```python
from build123d import *

# Parameters (mm, degrees)
F1_DEPTH = 67
F2_R     = 1.5
F3_DEPTH = 8
F4_R     = 1.875
F5_DEPTH = 9
F6_R     = 1.875
F7_DEPTH = 9
F8_R     = 1.875
F9_DEPTH = 9


# Not quite as in the source:
# - a feature names something its author has since deleted; it is built from what else it names


with BuildPart() as f1:
    # F0 (on Right) → F1 (new body)
    with BuildSketch(Plane.YZ):
        Polygon((14.9777059274, -37.1211464703), (14.9777059274, 53.8788535297), (8.9777059274, 53.8788535297), (8.9777059274, -31.1211464703), (5.4777059274, -31.1211464703), (5.4777059274, -16.1211464703), (-0.5222940726, -16.1211464703), (-0.5222940726, -37.1211464703), align=None)
    extrude(amount=F1_DEPTH)

    # F2 (on face) → F3 (join)
    with BuildSketch(Plane.YZ.offset(67)):
        with BuildLine():
            Line((11.9777059274, 43.8788535297), (11.9777059274, 45.3788535297))
            ThreePointArc((11.9777059274, 45.3788535297), (10.4777059274, 43.8788535297), (11.9777059274, 42.3788535297))
            Line((11.9777059274, 42.3788535297), (11.9777059274, 43.8788535297))
        make_face()
        with BuildLine():
            ThreePointArc((11.9777059274, 42.3788535297), (13.0383660992, 42.8181933579), (13.4777059274, 43.8788535297))
            ThreePointArc((13.4777059274, 43.8788535297), (13.0383660992, 44.9395137015), (11.9777059274, 45.3788535297))
            Line((11.9777059274, 45.3788535297), (11.9777059274, 43.8788535297))
            Line((11.9777059274, 43.8788535297), (11.9777059274, 42.3788535297))
        make_face()
        with BuildLine():
            ThreePointArc((13.4777059274, 23.8788535297), (13.0383660992, 24.9395137015), (11.9777059274, 25.3788535297))
            ThreePointArc((11.9777059274, 25.3788535297), (10.9170457557, 22.8181933579), (13.4777059274, 23.8788535297))
        make_face()
        with Locations((11.9777059274, -7.1211464703)):
            Circle(F2_R)
        with Locations((11.9777059274, -27.1211464703)):
            Circle(F2_R)
    extrude(amount=F3_DEPTH)

    # F4 (on face) → F5 (cut)
    with BuildSketch(Plane(origin=(0, 0, 0), x_dir=(0, -1, 0), z_dir=(-1, 0, 0))):
        with Locations((-18.4777059274, 23.8788535297)):
            Circle(F4_R)
        with Locations((-18.4777059274, 43.8788535297)):
            Circle(F4_R)
        with Locations((-18.4777059274, -7.1211464703)):
            Circle(F4_R)
        with Locations((-18.4777059274, -27.1211464703)):
            Circle(F4_R)
    extrude(amount=-F5_DEPTH, mode=Mode.SUBTRACT)

    # F6 (on face) → F7 (cut)
    with BuildSketch(Plane(origin=(0, 14.9777059274, 0), x_dir=(-1, 0, 0), z_dir=(0, 1, 0))):
        with Locations((-47, -34.1211464703)):
            Circle(F6_R)
        with Locations((-20, -34.1211464703)):
            Circle(F6_R)
    extrude(amount=-F7_DEPTH, mode=Mode.SUBTRACT)

    # F8 (on face) → F9 (cut)
    with BuildSketch(Plane(origin=(0, 0, 0), x_dir=(0, -1, 0), z_dir=(-1, 0, 0))):
        with BuildLine():
            ThreePointArc((-10.1027059274, 43.8788535297), (-10.6518807127, 45.2046787444), (-11.9777059274, 45.7538535297))
            Line((-11.9777059274, 45.7538535297), (-11.9777059274, 43.8788535297))
            Line((-11.9777059274, 43.8788535297), (-11.9777059274, 42.0038535297))
            ThreePointArc((-11.9777059274, 42.0038535297), (-10.6518807127, 42.553028315), (-10.1027059274, 43.8788535297))
        make_face()
        with BuildLine():
            ThreePointArc((-10.1027059274, 23.8788535297), (-10.6518807127, 25.2046787444), (-11.9777059274, 25.7538535297))
            ThreePointArc((-11.9777059274, 25.7538535297), (-13.3035311422, 22.553028315), (-10.1027059274, 23.8788535297))
        make_face()
        with BuildLine():
            Line((-11.9777059274, 43.8788535297), (-11.9777059274, 45.7538535297))
            ThreePointArc((-11.9777059274, 45.7538535297), (-13.8527059274, 43.8788535297), (-11.9777059274, 42.0038535297))
            Line((-11.9777059274, 42.0038535297), (-11.9777059274, 43.8788535297))
        make_face()
        with Locations((-11.9777059274, -27.1211464703)):
            Circle(F8_R)
        with Locations((-11.9777059274, -7.1211464703)):
            Circle(F8_R)
    extrude(amount=-F9_DEPTH, mode=Mode.SUBTRACT)


solid = f1.part
```
Geometry check sheet. Reference: the model listing, model coordinates, mm. A direction names the side the tool comes from. Give positions to 0.01 mm unless a question says otherwise; leave off trailing zeros. Order: outer loops, then holes, each group sorted by start corner. A loop starts at its lowest first (then second) coordinate and runs counter-clockwise, first axis right, second up. Notation, with made-up numbers: (-6.75, 57.5) - (29.25, 57.5) arc R18 ccw to (29.25, 63.5) - close; hole circle Ø8 at (17.25, 88.5). An arc over 180 degrees is marked (long way). Answer in a Markdown table with one row per item. Add a question column.
Q1. Cross-section at C-C, the plane x = 30. Enter the section's corners in (y, z).
Q2. Cross-section at D-D, the plane z = 21. Enter the section's corners in (x, y), then the cut area to 3 significant figures.
Q3. Tool access check on faces 4 (the flat face through (33, 3, -16.121)), 5 (the cylindrical face through (70.94, 12.67, -8.45)), 6 (the flat face through (33, 7, -31.121)), 7 (the flat face through (75, 12, -27)), 8 (the cylindrical face through (4.44, 10.19, -26.56)). Record the directions out of +Z, -Z, +X, -X, +Y, -Y that give a thin tool (end or side, any length) a straight path to the whole face; none if there is none.
Q4. Cross-section at A-A, the plane x = 20. Enter the section's corners in (y, z).
Q5. Mould release check, pull along X, two halves, no side actions. Record for faces 1 (the flat face through (33, 8.978, 12)), 2 (the flat face through (9, 12, -27)), 3 (the flat face through (47, 5.978, -34)): pulls with the +X half, pulls with the -X half, needs draft (parallel to the pull), parting line crosses it, or undercut.
Q6. Cross-section at B-B, the plane y = 4.25. Enter the section's corners in (x, z).
Q7. Material ranges on probe 1 along Y at (x, z) = (24, -24.5); probe 2 along Z at (x, y) = (44.5, 2.25); probe 3 along Y at (x, z) = (19.5, -6.5), recorded low to high. Write a range as from..to.
Q8. Gauge pin test, flat ends, axial feed: pin 1 (2.5 mm diameter, centred on y = 11.98, z = 23.88, fed in from -X); pin 2 (1.5 mm diameter, centred on x = 58, y = 5.5, fed in from +Z); pin 3 (4 mm diameter, centred on y = 9.5, z = 6.5, fed in from +X). Record the tip position at first contact, or that the pin passes through.
Check values:
| question | item | result |
|---|---|---|
| 1 | outline | (-0.52, -37.12) - (14.98, -37.12) - (14.98, 53.88) - (8.98, 53.88) - (8.98, -31.12) - (5.48, -31.12) - (5.48, -16.12) - (-0.52, -16.12) - close |
| 2 | outline | (0, 8.98) - (67, 8.98) - (67, 14.98) - (0, 14.98) - close |
| 2 | area | 402 mm^2 |
| 3 | face 4 | +Z, +X, -X, -Y |
| 3 | face 5 | +X |
| 3 | face 6 | +Z, +X, -X |
| 3 | face 7 | +Z, -Z, +X, +Y, -Y |
| 3 | face 8 | -X |
| 4 | outline | (-0.52, -37.12) - (14.98, -37.12) - (14.98, -36) - (5.98, -36) - (5.98, -32.25) - (14.98, -32.25) - (14.98, 53.88) - (8.98, 53.88) - (8.98, -31.12) - (5.48, -31.12) - (5.48, -16.12) - (-0.52, -16.12) - close |
| 5 | face 1 | needs draft |
| 5 | face 2 | pulls with the -X half |
| 5 | face 3 | undercut |
| 6 | outline | (0, -37.12) - (67, -37.12) - (67, -16.12) - (0, -16.12) - close |
| 7 | probe 1 | y = -0.52..5.48, 8.98..14.98 |
| 7 | probe 2 | z = -37.12..-16.12 |
| 7 | probe 3 | y = 8.98..14.98 |
| 8 | pin 1 | stops at x = 9 |
| 8 | pin 2 | stops at z = -16.12 |
| 8 | pin 3 | stops at x = 67 |
